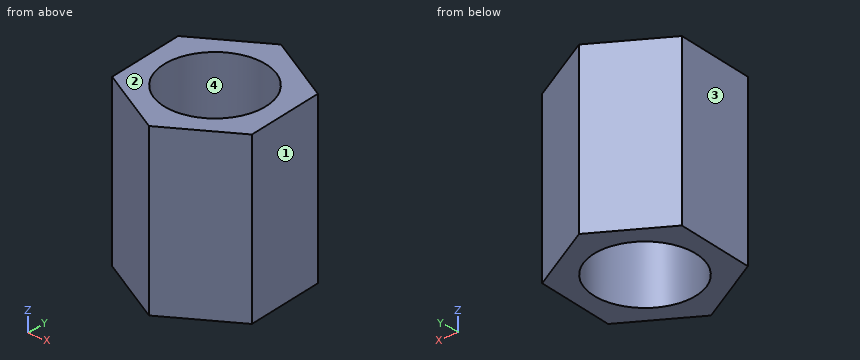
from build123d import *

# Parameters (mm, degrees)
F2_DEPTH = 22.5
F3_R     = 6.75
F4_DEPTH = 25


with BuildPart() as f2:
    # F0 (on Top) → F2 (new body)
    with BuildSketch(Plane.XY):
        Polygon((-0.505125, 10.669029), (-9.492213, 4.897064), (-8.987088, -5.771965), (0.505125, -10.669029), (9.492213, -4.897064), (8.987088, 5.771965), align=None)
    extrude(amount=F2_DEPTH)

    # F3 (on face) → F4 (cut)
    with BuildSketch(Plane.XY):
        Circle(F3_R)
    extrude(amount=F4_DEPTH, mode=Mode.SUBTRACT)


solid = f2.part
Verification items for the finished model (mm, model axes). Face numbers are marked on the shaded views. Give positions to 0.01 mm unless a question says otherwise; leave off trailing zeros. Order: outer loops, then holes, each group sorted by start corner. A loop starts at its lowest first (then second) coordinate and runs counter-clockwise, first axis right, second up. Notation, with made-up numbers: M -32.5,-5.75 L -9.5,-5.75 A9 cw -9.5,4.25 Z; hole C -5,12.25 d10. An arc over 180 degrees is marked long. Answer as a JSON object with one key per item and string values. Group by question number.
1) Cross-section at B-B (x = 0). Enter the section's corners in (y, z).
2) Cross-section at A-A (z = 12). Enter the section's corners in (x, y).
3) Cross-section at D-D (x = -7.75). Enter the section's corners in (y, z).
4) Depth check by flat-ended pin: pin 1 Ø2 at (x, z) = (2.5, 15.5) entering from -Y; pin 2 Ø3 at (x, y) = (2.5, -3.5) entering from +Z; pin 3 Ø3 at (y, z) = (7.5, 18.5) entering from +X; pin 4 Ø2 at (y, z) = (0.5, 18) entering from +X. Enter the tip coordinate at first touch or a pass-through.
5) Mould release check, pull along Y, two halves, no side actions. Record for the marked faces 1, 2, 3 and 4: released by +Y, released by -Y, zero draft, split by the parting line, or undercut.
6) Scan lines: line 1 along X through (y, z) = (-3, 4.5); line 2 along X through (y, z) = (0, 13.25); line 3 along Y through (x, z) = (2.25, 16). Record each from-to range of solid material in increasing order. Write a range as [from, to].
7) Cross-section at C-C (y = 0). Enter the section's corners in (x, z), then the cut area to 3 significant figures.
Result sheet:
{
 "1": {"outline": "M -10.41,0 L -6.75,0 L -6.75,22.5 L -10.41,22.5 Z; M 6.75,0 L 10.41,0 L 10.41,22.5 L 6.75,22.5 Z"},
 "2": {"outline": "M -9.49,4.9 L -8.99,-5.77 L 0.51,-10.67 L 9.49,-4.9 L 8.99,5.77 L -0.51,10.67 Z; hole C 0,0 d13.5"},
 "3": {"outline": "M -6.41,0 L 6.02,0 L 6.02,22.5 L -6.41,22.5 Z"},
 "4": {"pin 1": "stops at y = -10.03", "pin 2": "passes through", "pin 3": "stops at x = 8.55", "pin 4": "stops at x = 9.28"},
 "5": {"face 1": "released by +Y", "face 2": "zero draft", "face 3": "released by -Y", "face 4": "undercut"},
 "6": {"line 1": "x = [-9.12, -6.05], [6.05, 9.4]", "line 2": "x = [-9.26, -6.75], [6.75, 9.26]", "line 3": "y = [-9.55, -6.36], [6.36, 9.25]"},
 "7": {"outline": "M -9.26,0 L -6.75,0 L -6.75,22.5 L -9.26,22.5 Z; M 6.75,0 L 9.26,0 L 9.26,22.5 L 6.75,22.5 Z", "area": "113 mm2"}
}
